Here's how the part is built. I have some questions about the finished solid (model axes, mm). A direction names the side the tool comes from. Round coordinates to 2 decimals unless told otherwise and drop trailing zeros. Loops run counter-clockwise (first coordinate to the right, second up) from the corner with the lowest first, then second, coordinate; pieces in that order, holes last. Notation, with made-up numbers: M -21,70.5 L 14,70.5 A5 cw 14,75.5 Z; hole C 69,38 d11. An arc over 180 degrees is marked long. Use a Markdown table: item, result.
from build123d import *

# Parameters (mm, degrees)
F1_DEPTH = 5
F4_SIZE  = 1.99999
F5_R     = 5.99999
F6_SIZE  = 4


# Not quite as in the source:
# - a fillet or chamfer is up to 0.001 mm smaller than in the source, because OpenCascade refuses the exact size


with BuildPart() as f1:
    # F0 (on Top) → F1 (new body, symmetric)
    with BuildSketch(Plane.XY):
        with BuildLine():
            ThreePointArc((3.8729833462, -1), (-0.5040171699, -3.9681187851), (-4, 0))
            Line((-4, 0), (-4, 1.5))
            Line((-4, 1.5), (-5, 1.5))
            Line((-5, 1.5), (-7, -2.5))
            Line((-7, -2.5), (-5, -2.5))
            Line((-5, -2.5), (-5, -6))
            Line((-5, -6), (6, -6))
            Line((6, -6), (6, 6))
            Line((6, 6), (-8.8090169944, 6))
            Line((-8.8090169944, 6), (-8.8090169944, 1))
            ThreePointArc((-8.8090169944, 1), (-12.8090169944, -3), (-16.8090169944, 1))
            Line((-16.8090169944, 1), (-17.8090169944, 1))
            Line((-17.8090169944, 1), (-17.8090169944, -5))
            Line((-17.8090169944, -5), (-8.8090169944, -5))
            Line((-8.8090169944, -5), (-5.5, -5))
            Line((-5.5, -5), (-5.5, -3))
            Line((-5.5, -3), (-7.8090169944, -3))
            Line((-7.8090169944, -3), (-5.3090169944, 2))
            Line((-5.3090169944, 2), (-3.4641016151, 2))
            ThreePointArc((-3.4641016151, 2), (0.5401815135, 3.9633576589), (3.8729833462, 1))
            Line((3.8729833462, 1), (5.5, 1))
            Line((5.5, 1), (5.5, -1))
            Line((5.5, -1), (3.8729833462, -1))
        make_face()
    extrude(amount=F1_DEPTH, both=True)

    # F2 (on Top) → F3 (revolve, cut)
    with BuildSketch(Plane.XY):
        Polygon((0, 0), (-4, 0), (-4, -3.5), (-2, -5.5), (-2, -6), (0, -6), align=None)
    revolve(axis=Axis((0, -2.25, 0), (0, -1, 0)), mode=Mode.SUBTRACT)

    # F4 (size 2 in the source; OpenCascade refuses exactly that, so slightly less here)
    f4_edges = [f1.edges().sort_by_distance(p)[0] for p in [
        (-5.5, -5, 0),
    ]]
    chamfer(f4_edges, length=F4_SIZE)

    # F5 (radius 6 in the source; OpenCascade refuses exactly that, so slightly less here)
    f5_edges = [f1.edges().sort_by_distance(p)[0] for p in [
        (-17.809017, -5, 0),
    ]]
    fillet(f5_edges, radius=F5_R)

    # F6
    f6_edges = [f1.edges().sort_by_distance(p)[0] for p in [
        (-8.809017, 6, 0),
    ]]
    chamfer(f6_edges, length=F6_SIZE)


solid = f1.part
1. Imagine slicing it at A-A, the plane x = 0. Write out the boundary of the cut face in (y, z), then the cut area to 4 significant figures.
Answer sheet:
| item | result |
|---|---|
| outline | M -6,-5 L -4,-5 L -4,-3.5 L -5.5,-2 L -6,-2 Z; M -6,2 L -5.5,2 L -4,3.5 L -4,5 L -6,5 Z; M 4,-5 L 6,-5 L 6,5 L 4,5 Z |
| area | 29.75 mm2 |
2. I need wall thicknesses on probe 1 along Z at (x, y) = (0, -5.7); probe 2 along X at (y, z) = (-5.8, 0); probe 3 along X at (y, z) = (0.75, -4) (3 decimals). Which ranges of each line are inside material? Lowest first, please. Write a range as from..to.
Answer sheet:
| item | result |
|---|---|
| probe 1 | -5..-2, 2..5 |
| probe 2 | -5..-2, 2..6 |
| probe 3 | -17.804..-16.801, -8.817..-5.934, -5.375..-4, 5.5..6 |
3. We'd pull the mould along Z, two halves only. Please class faces 4 (the face through (-5, -4, 0)), 5 (the face through (-3, -3, 5)), 6 (the face through (-4, -2, 0)): +Z half, -Z half, draft (parallel to the pull), parting line (faces both ways), or undercut.
Answer sheet:
| item | result |
|---|---|
| face 4 | draft |
| face 5 | +Z half |
| face 6 | undercut |
4. Imagine slicing it at B-B, the plane y = -1.25. Write out the boundary of the cut face in (x, z) (3 decimals), then the cut area to 3 significant figures.
Answer sheet:
| item | result |
|---|---|
| outline | M -17.371,-5 L -16.116,-5 L -16.116,5 L -17.371,5 Z; M -9.502,-5 L -6.934,-5 L -6.934,5 L -9.502,5 Z; M -6.375,-5 L -3.8,-5 L -3.8,-1.25 A4 cw -3.8,1.25 L -3.8,5 L -6.375,5 Z; M 3.8,-5 L 6,-5 L 6,5 L 3.8,5 L 3.8,1.25 A4 cw 3.8,-1.25 Z |
| area | 85.3 mm2 |
5. Imagine slicing it at D-D, the plane y = 0.5. Write out the boundary of the cut face in (x, z).
Answer sheet:
| item | result |
|---|---|
| outline | M -17.79,-5 L -16.78,-5 L -16.78,5 L -17.79,5 Z; M -8.84,-5 L -6.06,-5 L -6.06,5 L -8.84,5 Z; M -5.5,-5 L -4,-5 L -4,5 L -5.5,5 Z; M 5.5,-5 L 6,-5 L 6,5 L 5.5,5 Z |
6. Imagine slicing it at C-C, the plane x = -6. Write out the boundary of the cut face in (y, z), then the cut area to 3 significant figures.
Answer sheet:
| item | result |
|---|---|
| outline | M -3.5,-5 L -3,-5 L -3,5 L -3.5,5 Z; M -2.5,-5 L -0.5,-5 L -0.5,5 L -2.5,5 Z; M 0.62,-5 L 4.81,-5 L 4.81,5 L 0.62,5 Z |
| area | 66.9 mm2 |
7. Which directions (+Z, -Z, +X, -X, +Y, -Y) give clear straight access to the entire face, cutting with the end or side of a thin tool? Please do faces 1 (the face through (0, 4, 0)), 2 (the face through (-17, 1, 0)), 3 (the face through (-10, -5, 0)).
Answer sheet:
| item | result |
|---|---|
| face 1 | +Z, -Z |
| face 2 | +Z, -Z, -X, +Y |
| face 3 | +Z, -Z, -X, -Y |
8. For pin 1 Ø0.7 at (x, z) = (-6.5, 2) entering from +Y; pin 2 Ø1.6 at (y, z) = (-0.5, 0) entering from -X; pin 3 Ø0.8 at (x, z) = (-17, -1) entering from +Y, each with a flat end and sliding along its axis, tell me the tip position at first contact or that it passes through.
Answer sheet:
| item | result |
|---|---|
| pin 1 | y = 4.66 |
| pin 2 | x = -17.77 |
| pin 3 | y = 1 |
